For this review, take the finished solid that the model builds, in its own axes (mm). Face numbers are marked on the shaded views. A direction names the side the tool comes from. Give positions to 0.01 mm unless a question says otherwise; leave off trailing zeros. Write each loop counter-clockwise with the first axis right and the second up, starting at its lowest first coordinate (ties: lowest second). Pieces come first, ordered by that corner, then holes. Notation, with made-up numbers: M -28.75,12.5 L 19.25,12.5 A14 ccw 19.25,18.5 Z; hole C 20.25,20.5 d2. An arc over 180 degrees is marked long. Use one line per item in the form item = value. Start each with the question number.
Q1. Tool access review of the marked faces 1 and 2: name each direction out of +Z, -Z, +X, -X, +Y, -Y from which nothing blocks a thin tool from reaching the whole face with its end or side.
Q2. Mouldability with a two-part tool opening along X and no side actions: class the marked faces 3, 4 and 5 as released by +X, released by -X, zero draft, split by the parting line, or undercut.
Q3. Consider section B-B on y = 22.5. Write out the cut boundary in (x, z).
Q4. Consider section C-C on x = -14. Write out the cut boundary in (y, z), and give its area (3 significant figures).
Q5. Consider section A-A on z = 24.5. Write out the cut boundary in (x, y), and give its area (3 significant figures).
Q6. Clearance check with a flat-ended pin moving along its axis: pin 1 Ø7.5 at (x, y) = (0.5, 15) entering from +Z. State where the tip first meets the part, or that it passes through.
Q7. For probe 1 along X at (y, z) = (23.75, 24); probe 2 along Z at (x, y) = (-12, 20.25), list the stretches that pass through material, from the lowest coordinate up. Write a range as [from, to].
```python
from build123d import *

# Parameters (mm, degrees)
BOSS_EXTRUDE1_DEPTH     = 10
SKETCH2_W               = 17.2
SKETCH2_H               = 43
CUT_EXTRUDE1_DEPTH      = 72.414284285
SKETCH3_W               = 90
SKETCH3_H               = 34
SKETCH3_W_2             = 80
SKETCH3_H_2             = 24
BOSS_EXTRUDE3_DEPTH     = 15
SKETCH4_W               = 49.6
SKETCH4_H               = 5
BOSS_EXTRUDE4_DEPTH     = 10
SKETCH5_W               = 15
SKETCH5_H               = 22
BOSS_EXTRUDE5_DEPTH     = 5
SKETCH6_W               = 90
SKETCH6_H               = 77
BOSS_EXTRUDE6_DEPTH     = 15
BOSS_EXTRUDE8_DEPTH     = 39
CHAMFER1_SIZE           = 64
CHAMFER1_SIZE_2         = 3.354097874
CHAMFER2_SIZE           = 64
CHAMFER2_SIZE_2         = 11.405813635
CHAMFER3_SIZE           = 64
CHAMFER3_SIZE_2         = 13.775745352
CUT_EXTRUDE3_DEPTH      = 95.500525601
CUT_EXTRUDE3_DEPTH_BACK = 95.500525601
SKETCH10_W              = 50
SKETCH10_H              = 27
SKETCH11_W              = 45.5
SKETCH11_H              = 10.5
CUT_EXTRUDE4_DEPTH      = 7.5
SKETCH14_W              = 2.05
SKETCH14_H              = 10.5
BOSS_EXTRUDE9_DEPTH     = 15
SKETCH15_R              = 8
CUT_EXTRUDE5_DEPTH      = 122.227059686
CUT_EXTRUDE6_DEPTH      = 2.5
CUT_EXTRUDE7_REACH      = 97.373
SKETCH18_W              = 29.6
SKETCH18_H              = 45
CUT_EXTRUDE8_DEPTH      = 15
SKETCH21_W              = 29.6
SKETCH21_H              = 15
BOSS_EXTRUDE10_DEPTH    = 2.5
SKETCH22_OUTSIDE_W      = 133.046
SKETCH22_OUTSIDE_H      = 133.046
SKETCH22_OUTSIDE_W_2    = 90
SKETCH22_OUTSIDE_H_2    = 72
CUT_EXTRUDE9_DEPTH      = 64
CUT_EXTRUDE10_DEPTH     = 10


with BuildPart() as part:
    # Sketch1 → Boss-Extrude1 (new body)
    with BuildSketch(Plane(origin=(0, 0, 0), x_dir=(1, 0, 0), z_dir=(0, 1, 0))):
        with BuildLine():
            Line((-35, 50), (35, 50))
            ThreePointArc((35, 50), (45.606601718, 45.606601718), (50, 35))
            Line((50, 35), (50, -35))
            ThreePointArc((50, -35), (45.606601718, -45.606601718), (35, -50))
            Line((35, -50), (-35, -50))
            ThreePointArc((-35, -50), (-45.606601718, -45.606601718), (-50, -35))
            Line((-50, -35), (-50, 35))
            ThreePointArc((-50, 35), (-45.606601718, 45.606601718), (-35, 50))
        make_face()
    extrude(amount=BOSS_EXTRUDE1_DEPTH)

    # Sketch2 → Cut-Extrude1 (cut, through all)
    with BuildSketch(Plane(origin=(0, 10, 0), x_dir=(1, 0, 0), z_dir=(0, 1, 0))):
        with Locations((-33.4, 18.5)):
            Rectangle(SKETCH2_W, SKETCH2_H)
        with Locations((33.4, 18.5)):
            Rectangle(SKETCH2_W, SKETCH2_H)
    extrude(amount=-CUT_EXTRUDE1_DEPTH, mode=Mode.SUBTRACT)

    # Sketch3 → Boss-Extrude3 (add)
    with BuildSketch(Plane(origin=(0, 10, 0), x_dir=(1, 0, 0), z_dir=(0, 1, 0))):
        with Locations((0, -20)):
            Rectangle(SKETCH3_W, SKETCH3_H)
        with Locations((0, -20)):
            Rectangle(SKETCH3_W_2, SKETCH3_H_2, mode=Mode.SUBTRACT)
    extrude(amount=BOSS_EXTRUDE3_DEPTH)

    # Sketch4 → Boss-Extrude4 (add)
    with BuildSketch(Plane(origin=(0, 10, 0), x_dir=(1, 0, 0), z_dir=(0, 1, 0))):
        with Locations((0, 10)):
            Rectangle(SKETCH4_W, SKETCH4_H)
        with Locations((0, 27)):
            Rectangle(SKETCH4_W, SKETCH4_H)
    extrude(amount=BOSS_EXTRUDE4_DEPTH)

    # Sketch5 → Boss-Extrude5 (add)
    with BuildSketch(Plane(origin=(0, 20, 0), x_dir=(1, 0, 0), z_dir=(0, 1, 0))):
        with Locations((-17.3, 18.5)):
            Rectangle(SKETCH5_W, SKETCH5_H)
        with Locations((17.3, 18.5)):
            Rectangle(SKETCH5_W, SKETCH5_H)
    extrude(amount=BOSS_EXTRUDE5_DEPTH)

    # Sketch6 → Boss-Extrude6 (add)
    with BuildSketch(Plane(origin=(0, 10, 0), x_dir=(1, 0, 0), z_dir=(0, 1, 0))):
        with BuildLine():
            Line((-50, 35), (-50, -35))
            ThreePointArc((-50, -35), (-45.606601718, -45.606601718), (-35, -50))
            Line((-35, -50), (35, -50))
            ThreePointArc((35, -50), (45.606601718, -45.606601718), (50, -35))
            Line((50, -35), (50, 35))
            ThreePointArc((50, 35), (45.606601718, 45.606601718), (35, 50))
            Line((35, 50), (-35, 50))
            ThreePointArc((-35, 50), (-45.606601718, 45.606601718), (-50, 35))
        make_face()
        with Locations((0, 1.5)):
            Rectangle(SKETCH6_W, SKETCH6_H, mode=Mode.SUBTRACT)
    extrude(amount=BOSS_EXTRUDE6_DEPTH)

    # Sketch9 → Boss-Extrude8 (add)
    with BuildSketch(Plane(origin=(0, 25, 0), x_dir=(1, 0, 0), z_dir=(0, 1, 0))):
        with BuildLine():
            Line((-50, 35), (-50, -35))
            ThreePointArc((-50, -35), (-45.606601718, -45.606601718), (-35, -50))
            Line((-35, -50), (35, -50))
            ThreePointArc((35, -50), (45.606601718, -45.606601718), (50, -35))
            Line((50, -35), (50, 35))
            ThreePointArc((50, 35), (45.606601718, 45.606601718), (35, 50))
            Line((35, 50), (-35, 50))
            ThreePointArc((-35, 50), (-45.606601718, 45.606601718), (-50, 35))
        make_face()
        with BuildLine():
            Line((-45, 35), (-45, -32))
            Line((-45, -32), (45, -32))
            Line((45, -32), (45, 35))
            ThreePointArc((45, 35), (44.659258263, 37.588190451), (43.660254038, 40))
            Line((43.660254038, 40), (-43.660254038, 40))
            ThreePointArc((-43.660254038, 40), (-44.659258263, 37.588190451), (-45, 35))
        make_face(mode=Mode.SUBTRACT)
    extrude(amount=BOSS_EXTRUDE8_DEPTH)

    # Chamfer1
    # the kernel refuses this chamfer: 64, 3.354097874 mm, written as the material it takes off along each edge
    with BuildSketch(Plane(origin=(-35, 64, 50), x_dir=(0, -0.9999979738662979, 0.002013023422382214), z_dir=(1, 0, 0)), Plane(origin=(50, 64, 35), x_dir=(0.002013023422382214, -0.9999979738662979, 0), z_dir=(0, 0, -1)), Plane(origin=(-50, 64, -35), x_dir=(-0.002013023422382214, -0.9999979738662979, 0), z_dir=(0, 0, 1)), Plane(origin=(35, 64, -50), x_dir=(0, -0.9999979738662979, -0.002013023422382214), z_dir=(-1, 0, 0))) as chamfer1_piece_1:
        Polygon((CHAMFER1_SIZE * 0.999997973866, CHAMFER1_SIZE * 0.00201302342238), (-CHAMFER1_SIZE_2 * 0.00201302342245, CHAMFER1_SIZE_2 * 0.9999979739), (0, 0), align=None)
    extrude(amount=70, mode=Mode.SUBTRACT)
    with BuildSketch(Plane(origin=(35, 64, 35), x_dir=(0, 0, 1), z_dir=(-1, 0, 0))) as chamfer1_piece_2:
        Polygon((15, -CHAMFER1_SIZE), (15 - CHAMFER1_SIZE_2, 0), (15, 0), align=None)
    revolve(axis=Axis((35, 64, 35), (0, 1, 0)), revolution_arc=90, mode=Mode.SUBTRACT)
    with BuildSketch(Plane(origin=(-35, 64, 35), x_dir=(-1, 0, 0), z_dir=(0, 0, -1))) as chamfer1_piece_3:
        Polygon((15, -CHAMFER1_SIZE), (15 - CHAMFER1_SIZE_2, 0), (15, 0), align=None)
    revolve(axis=Axis((-35, 64, 35), (0, 1, 0)), revolution_arc=90, mode=Mode.SUBTRACT)
    with BuildSketch(Plane(origin=(35, 64, -35), x_dir=(1, 0, 0), z_dir=(0, 0, 1))) as chamfer1_piece_4:
        Polygon((15, -CHAMFER1_SIZE), (15 - CHAMFER1_SIZE_2, 0), (15, 0), align=None)
    revolve(axis=Axis((35, 64, -35), (0, 1, 0)), revolution_arc=90, mode=Mode.SUBTRACT)
    with BuildSketch(Plane(origin=(-35, 64, -35), x_dir=(0, 0, -1), z_dir=(1, 0, 0))) as chamfer1_piece_5:
        Polygon((15 - CHAMFER1_SIZE_2, 0), (15, -CHAMFER1_SIZE), (15, 0), align=None)
    revolve(axis=Axis((-35, 64, -35), (0, 1, 0)), revolution_arc=90, mode=Mode.SUBTRACT)

    # Chamfer2
    # the kernel refuses this chamfer: 64, 11.405813635 mm, written as the material it takes off along each edge
    with BuildSketch(Plane(origin=(201.306482971, 64, -46.645902126), x_dir=(0, -0.9982575003065525, -0.05900816114499234), z_dir=(-1, 0, 0))) as chamfer2_piece_1:
        Polygon((CHAMFER2_SIZE * 0.999977671636, CHAMFER2_SIZE * 0.0066825316561), (-CHAMFER2_SIZE_2 * 0.0590081611462, CHAMFER2_SIZE_2 * 0.998257500326), (0, 0), align=None)
    extrude(amount=402.612965942, mode=Mode.SUBTRACT)

    # Chamfer3
    # the kernel refuses this chamfer: 64, 13.775745352 mm, written as the material it takes off along each edge
    with BuildSketch(Plane(origin=(-201.265469314, 64, 46.645902126), x_dir=(0, -0.9981787050157903, 0.06032638604292662), z_dir=(1, 0, 0))) as chamfer3_piece_1:
        Polygon((CHAMFER3_SIZE * 0.999967974892, CHAMFER3_SIZE * 0.00800307379952), (-CHAMFER3_SIZE_2 * 0.060326386045, CHAMFER3_SIZE_2 * 0.99817870505), (0, 0), align=None)
    extrude(amount=402.530938629, mode=Mode.SUBTRACT)

    # Sketch10 → Cut-Extrude3 (cut, two sides: drawn at the far end of the back side and taken through both)
    with BuildSketch(Plane(origin=(0, 1.307501734, 0), x_dir=(0, 0, 1), z_dir=(-1, 0, 0)).offset(-CUT_EXTRUDE3_DEPTH_BACK)):
        with Locations((-22.129843227, 49.192498266)):
            Rectangle(SKETCH10_W, SKETCH10_H)
    extrude(amount=CUT_EXTRUDE3_DEPTH + CUT_EXTRUDE3_DEPTH_BACK, mode=Mode.SUBTRACT)

    # Sketch11 → Cut-Extrude4 (cut)
    with BuildSketch(Plane(origin=(0, 10, 0), x_dir=(1, 0, 0), z_dir=(0, 1, 0))):
        with Locations((0, 34.75)):
            Rectangle(SKETCH11_W, SKETCH11_H)
    extrude(amount=-CUT_EXTRUDE4_DEPTH, mode=Mode.SUBTRACT)

    # Sketch14 → Boss-Extrude9 (add)
    with BuildSketch(Plane(origin=(0, 10, 0), x_dir=(1, 0, 0), z_dir=(0, 1, 0))):
        with Locations((-23.775, 34.75)):
            Rectangle(SKETCH14_W, SKETCH14_H)
        with Locations((23.775, 34.75)):
            Rectangle(SKETCH14_W, SKETCH14_H)
    extrude(amount=BOSS_EXTRUDE9_DEPTH)

    # Sketch15 → Cut-Extrude5 (cut, through all)
    with BuildSketch(Plane.XY.offset(-40)):
        with Locations((-12.75, 12.75)):
            Circle(SKETCH15_R)
        with Locations((12.75, 12.75)):
            Circle(SKETCH15_R)
    extrude(amount=-CUT_EXTRUDE5_DEPTH, mode=Mode.SUBTRACT)

    # Sketch17 → Cut-Extrude6 (cut)
    with BuildSketch(Plane(origin=(0, 0, -29.5), x_dir=(-1, 0, 0), z_dir=(0, 0, -1))):
        Polygon((-9.8, 25), (-22.75, 25), (-22.75, 2.5), (22.75, 2.5), (22.75, 25), (9.8, 25), (9.8, 20), (-9.8, 20), align=None)
    extrude(amount=-CUT_EXTRUDE6_DEPTH, mode=Mode.SUBTRACT)

    # Cut-Extrude7: up to this face of the body (flat: up to its plane)
    cut_extrude7_end = Plane(part.part.faces().sort_by_distance((0, 10, -18.5))[0])
    # Sketch18 → Cut-Extrude7 (cut, up to the picked face)
    with BuildSketch(Plane.XZ, mode=Mode.PRIVATE) as cut_extrude7_sk1:
        with Locations((0, -4.5)):
            Rectangle(SKETCH18_W, SKETCH18_H)
    cut_extrude7_tool1 = split(extrude(cut_extrude7_sk1.sketch, amount=-CUT_EXTRUDE7_REACH, mode=Mode.PRIVATE), bisect_by=cut_extrude7_end, keep=Keep.BOTH, mode=Mode.PRIVATE)
    add(cut_extrude7_tool1.solids().sort_by(Axis((0, 0, -4.5), (0, 1, 0)))[0], mode=Mode.SUBTRACT)

    # Sketch20 → Cut-Extrude8 (cut)
    with BuildSketch(Plane.XZ.offset(-25)):
        with BuildLine():
            Line((-45, -35), (-45, -40))
            Line((-45, -40), (-43.660254038, -40))
            ThreePointArc((-43.660254038, -40), (-44.659258263, -37.588190451), (-45, -35))
        make_face()
        with BuildLine():
            Line((45, -40), (45, -35))
            ThreePointArc((45, -35), (44.659258263, -37.588190451), (43.660254038, -40))
            Line((43.660254038, -40), (45, -40))
        make_face()
    extrude(amount=-CUT_EXTRUDE8_DEPTH, mode=Mode.SUBTRACT)

    # Sketch21 → Boss-Extrude10 (add)
    with BuildSketch(Plane.XZ):
        with Locations((0, -4.5)):
            Rectangle(SKETCH21_W, SKETCH21_H)
    extrude(amount=-BOSS_EXTRUDE10_DEPTH)

    # Sketch22 outside → Cut-Extrude9 (cut)
    with BuildSketch(Plane(origin=(0, 64, 0), x_dir=(1, 0, 0), z_dir=(0, 1, 0))):
        Rectangle(SKETCH22_OUTSIDE_W, SKETCH22_OUTSIDE_H)
        with Locations((0, 4)):
            Rectangle(SKETCH22_OUTSIDE_W_2, SKETCH22_OUTSIDE_H_2, mode=Mode.SUBTRACT)
    extrude(amount=-CUT_EXTRUDE9_DEPTH, mode=Mode.SUBTRACT)

    # Sketch23 → Cut-Extrude10 (cut)
    with BuildSketch(Plane.XZ):
        Polygon((-24.8, 3), (-24.8, -40), (24.8, -40), (24.8, 3), (42, 3), (42, -40), (45, -40), (45, 32), (-45, 32), (-45, -40), (-42, -40), (-42, 3), align=None)
    extrude(amount=-CUT_EXTRUDE10_DEPTH, mode=Mode.SUBTRACT)


with BuildPart() as cut_extrude10_piece_1:
    # of the separate pieces the step leaves, piece 1, a body of its own (cut_extrude10_pieces)
    add(part.part.solids().sort_by_distance((45, 10, 3))[0])


with BuildPart() as cut_extrude10_piece_2:
    # of the separate pieces the step leaves, piece 2, a body of its own (cut_extrude10_pieces)
    add(part.part.solids().sort_by_distance((24.8, 25, -7.5))[0])


solid = cut_extrude10_piece_1.part
```
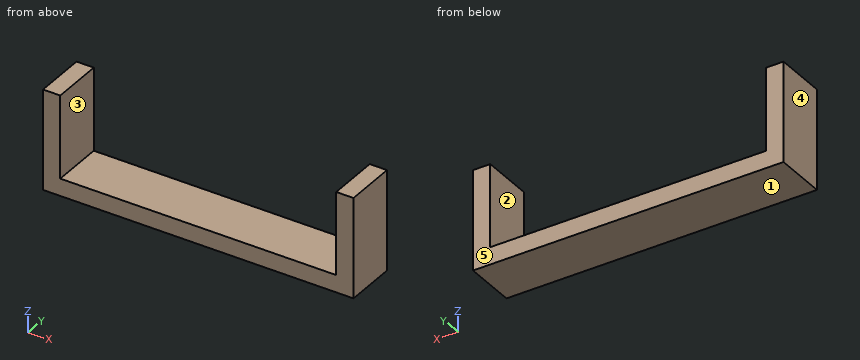
Working result:
q1.face_1 = -Z, +X, -X, +Y, -Y
q1.face_2 = +Z, +Y, -Y
q2.face_3 = undercut
q2.face_4 = released by -X
q2.face_5 = zero draft
q3.outline = M -45,3 L 45,3 L 45,32 L 40,32 L 40,8 L -40,8 L -40,32 L -45,32 Z
q4.outline = M 10,3 L 25,3 L 25,8 L 10,8 Z
q4.area = 75.0 mm²
q5.outline = M -45,10 L -40,10 L -40,25 L -45,25 Z; M 40,10 L 45,10 L 45,25 L 40,25 Z
q5.area = 150 mm²
q6.pin_1 = 8
q7.probe_1 = [-45, -40], [40, 45]
q7.probe_2 = [3, 8]
